The figure shows three views and two pictorial views of one solid part (mm, origin at its lowest corner). Answer the questions. A direction names the side the tool comes from. Give positions to 0.01 mm unless a question says otherwise; leave off trailing zeros. Order: outer loops, then holes, each group sorted by start corner. A loop starts at its lowest first (then second) coordinate and runs counter-clockwise, first axis right, second up. Notation, with made-up numbers: M 33,75 L 48,75 A22 cw 48,112 Z; hole C 25,-31.75 d6. An arc over 180 degrees is marked long. One line per item, written item: value.
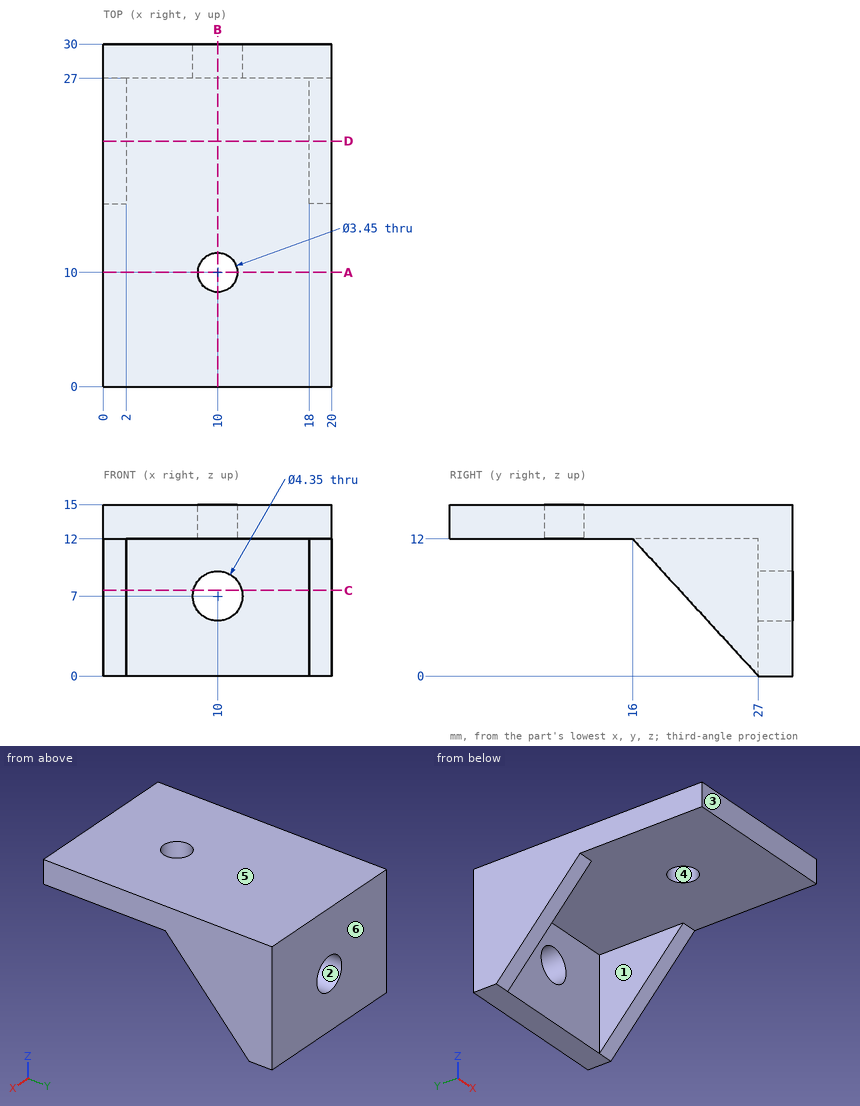
1) Consider probe 1 along X at (y, z) = (27.8, 7) (3 decimals); probe 2 along Y at (x, z) = (10, 13.1) (3 decimals); probe 3 along X at (y, z) = (20.75, 11.5). Determine where each line is inside the solid, lowest interval first.
Reported:
probe 1: x = 0 to 7.825, 12.175 to 20
probe 2: y = 0 to 8.275, 11.725 to 30
probe 3: x = 0 to 2, 18 to 20
2) Find section B-B, the plane x = 10. Write down the section's boundary in (y, z) (3 decimals).
Reported:
outline: M 0,12 L 8.275,12 L 8.275,15 L 0,15 Z; M 11.725,12 L 27,12 L 27,9.175 L 30,9.175 L 30,15 L 11.725,15 Z; M 27,0 L 30,0 L 30,4.825 L 27,4.825 Z
3) Find section C-C, the plane z = 7.5. Write down the section's boundary in (x, y) (3 decimals), plus the area to 3 significant figures.
Reported:
outline: M 0,20.125 L 2,20.125 L 2,27 L 7.883,27 L 7.883,30 L 0,30 Z; M 12.117,27 L 18,27 L 18,20.125 L 20,20.125 L 20,30 L 12.117,30 Z
area: 74.8 mm^2
4) Each of these flat-tipped pins is pushed along its axis until it touches: pin 1 Ø2 at (x, y) = (10, 10) entering from -Z; pin 2 Ø3 at (x, z) = (16, 7) entering from -Y; pin 3 Ø10 at (x, y) = (10, 13) entering from -Z. Where does it stop, or does it pass through?
Reported:
pin 1: passes through
pin 2: stops at y = 27
pin 3: stops at z = 12
5) Which of the six approach directions +Z, -Z, +X, -X, +Y, -Y give full straight-line access (tool end or side, diameter ignored) to the marked faces 1 and 2?
Reported:
face 1: -Z, -Y
face 2: +Y, -Y
6) Find section A-A, the plane y = 10. Write down the section's boundary in (x, z) (3 decimals), plus the area to 4 significant figures.
Reported:
outline: M 0,12 L 8.275,12 L 8.275,15 L 0,15 Z; M 11.725,12 L 20,12 L 20,15 L 11.725,15 Z
area: 49.65 mm^2
7) Find section D-D, the plane y = 21.5. Write down the section's boundary in (x, z), plus the area to 3 significant figures.
Reported:
outline: M 0,6 L 2,6 L 2,12 L 18,12 L 18,6 L 20,6 L 20,15 L 0,15 Z
area: 84.0 mm^2
8) Determine the mould class of the marked faces 3, 4, 5 and 6 for opening direction Y: +Y half, -Y half, draft (parallel to the pull), parting line (faces both ways), or undercut.
Reported:
face 3: -Y half
face 4: undercut
face 5: draft
face 6: +Y half
